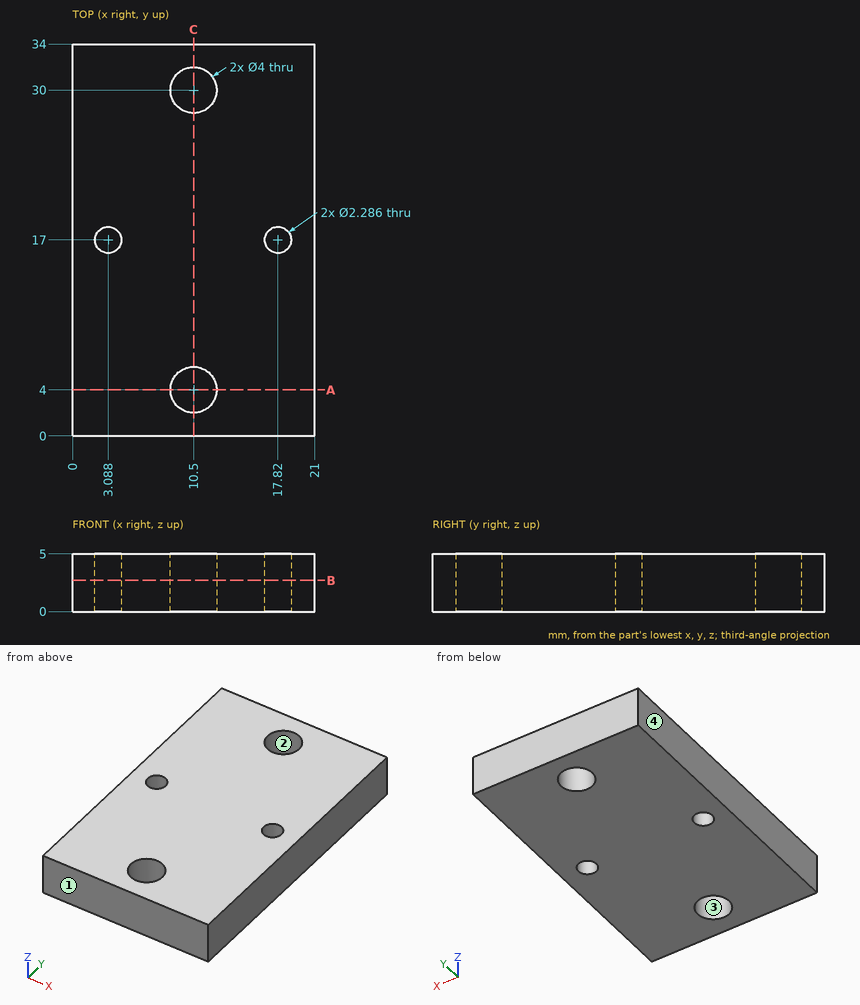
Geometry check sheet. Reference: drawing and pictorial views, mm from the part's lowest x, y, z. Give positions to 0.01 mm unless a question says otherwise; leave off trailing zeros. Write each loop counter-clockwise with the first axis right and the second up, starting at its lowest first coordinate (ties: lowest second). Pieces come first, ordered by that corner, then holes. Notation, with made-up numbers: (16.25, -20.5) - (34.25, -20.5) arc R10 cw to (34.25, -16.5) - close; hole circle Ø2 at (67, 72.5). An arc over 180 degrees is marked (long way). Use a Markdown table: item, result.
Q1. Go/stop test with a flat-tipped pin: P1, Ø2, axis at x = 3.09, y = 17, coming from the +Z side. Record where the tip stops, or that it passes through.
Computed:
| item | result |
|---|---|
| P1 | passes through |
Q2. Section check B-B, the plane z = 2.7. Enter the section's corners in (x, y) (1 decimal), then the cut area to 3 significant figures.
Computed:
| item | result |
|---|---|
| outline | (0, 0) - (21, 0) - (21, 34) - (0, 34) - close; hole circle Ø2.3 at (3.1, 17); hole circle Ø4 at (10.5, 4); hole circle Ø4 at (10.5, 30); hole circle Ø2.3 at (17.8, 17) |
| area | 681 mm² |
Q3. Thickness scan on L1, parallel to Y at x = 10.5, z = 3; L2, parallel to Y at x = 10, z = 2.65 (1 decimal); L3, parallel to X at y = 18, z = 4.05 (1 decimal). Record the ranges inside material, lowest first. Write a range as [from, to].
Computed:
| item | result |
|---|---|
| L1 | y = [0, 2], [6, 28], [32, 34] |
| L2 | y = [0, 2.1], [5.9, 28.1], [31.9, 34] |
| L3 | x = [0, 2.5], [3.6, 17.3], [18.4, 21] |
Q4. Draft check along X on the marked faces 1, 2, 3 and 4. Enter one of: pulls with the +X half, pulls with the -X half, needs draft (parallel to the pull), parting line crosses it, or undercut.
Computed:
| item | result |
|---|---|
| face 1 | needs draft |
| face 2 | undercut |
| face 3 | undercut |
| face 4 | pulls with the -X half |
Q5. Section check C-C, the plane x = 10.5. Enter the section's corners in (y, z), then the cut area to 3 significant figures.
Computed:
| item | result |
|---|---|
| outline | (0, 0) - (2, 0) - (2, 5) - (0, 5) - close; (6, 0) - (28, 0) - (28, 5) - (6, 5) - close; (32, 0) - (34, 0) - (34, 5) - (32, 5) - close |
| area | 130 mm² |
Q6. Section check A-A, the plane y = 4. Enter the section's corners in (x, z).
Computed:
| item | result |
|---|---|
| outline | (0, 0) - (8.5, 0) - (8.5, 5) - (0, 5) - close; (12.5, 0) - (21, 0) - (21, 5) - (12.5, 5) - close |
